from build123d import *

# Parameters (mm, degrees)
SKETCH1_W               = 297
SKETCH1_H               = 210
BOSS_EXTRUDE1_DEPTH     = 3
SKETCH2_OUTSIDE_W       = 371.752
SKETCH2_OUTSIDE_H       = 284.752
SKETCH2_OUTSIDE_R       = 1.5
LASER_CUT_PROFILE_DEPTH = 364.755412331


with BuildPart() as part:
    # Sketch1 → Boss-Extrude1 (new body)
    with BuildSketch(Plane(origin=(0, 0, 0), x_dir=(1, 0, 0), z_dir=(0, 1, 0))):
        with Locations((148.5, 105)):
            Rectangle(SKETCH1_W, SKETCH1_H)
    extrude(amount=BOSS_EXTRUDE1_DEPTH)

    # Sketch2 outside → Laser Cut Profile (cut, through all)
    # profile 1 of 14: a face of its own
    with BuildSketch(Plane(origin=(0, 3, 0), x_dir=(1, 0, 0), z_dir=(0, 1, 0))):
        with Locations((148.5, 105)):
            Rectangle(SKETCH2_OUTSIDE_W, SKETCH2_OUTSIDE_H)
        with BuildLine():
            Line((5, 2), (292, 2))
            ThreePointArc((292, 2), (294.121320344, 2.878679656), (295, 5))
            Line((295, 5), (295, 125))
            ThreePointArc((295, 125), (294.712859503, 126.280778403), (293.906404455, 127.316381241))
            Line((293.906404455, 127.316381241), (228.29357677, 181.316381241))
            ThreePointArc((228.29357677, 181.316381241), (227.399806572, 181.823928445), (226.387172315, 182))
            Line((226.387172315, 182), (70.612827685, 182))
            ThreePointArc((70.612827685, 182), (69.600193428, 181.823928445), (68.70642323, 181.316381241))
            Line((68.70642323, 181.316381241), (3.093595545, 127.316381241))
            ThreePointArc((3.093595545, 127.316381241), (2.287140497, 126.280778403), (2, 125))
            Line((2, 125), (2, 5))
            ThreePointArc((2, 5), (2.878679656, 2.878679656), (5, 2))
        make_face(mode=Mode.SUBTRACT)
    # profile 2 of 14: a face of its own
    with BuildSketch(Plane(origin=(0, 3, 0), x_dir=(1, 0, 0), z_dir=(0, 1, 0))):
        with Locations(Location((93.3, 92.8, 0), (0, 0, 270))):
            Circle(SKETCH2_OUTSIDE_R)
    # profile 3 of 14: a face of its own
    with BuildSketch(Plane(origin=(0, 3, 0), x_dir=(1, 0, 0), z_dir=(0, 1, 0))):
        with Locations(Location((141.2, 98.9, 0), (0, 0, 270))):
            Circle(SKETCH2_OUTSIDE_R)
    # profile 4 of 14: a face of its own
    with BuildSketch(Plane(origin=(0, 3, 0), x_dir=(1, 0, 0), z_dir=(0, 1, 0))):
        with Locations(Location((136.2, 68.95, 0), (0, 0, 270))):
            Circle(SKETCH2_OUTSIDE_R)
    # profile 5 of 14: a face of its own
    with BuildSketch(Plane(origin=(0, 3, 0), x_dir=(1, 0, 0), z_dir=(0, 1, 0))):
        with Locations(Location((108.5, 68.95, 0), (0, 0, 270))):
            Circle(SKETCH2_OUTSIDE_R)
    # profile 6 of 14: a face of its own
    with BuildSketch(Plane(origin=(0, 3, 0), x_dir=(1, 0, 0), z_dir=(0, 1, 0))):
        with Locations(Location((93.2, 18.35, 0), (0, 0, 270))):
            Circle(SKETCH2_OUTSIDE_R)
    # profile 7 of 14: a face of its own
    with BuildSketch(Plane(origin=(0, 3, 0), x_dir=(1, 0, 0), z_dir=(0, 1, 0))):
        with Locations(Location((141.2, 17.1, 0), (0, 0, 270))):
            Circle(SKETCH2_OUTSIDE_R)
    # profile 8 of 14: a face of its own
    with BuildSketch(Plane(origin=(0, 3, 0), x_dir=(1, 0, 0), z_dir=(0, 1, 0))):
        with Locations(Location((151.6, 18.4, 0), (0, 0, 270))):
            Circle(SKETCH2_OUTSIDE_R)
    # profile 9 of 14: a face of its own
    with BuildSketch(Plane(origin=(0, 3, 0), x_dir=(1, 0, 0), z_dir=(0, 1, 0))):
        with Locations(Location((166.65, 68.9, 0), (0, 0, 270))):
            Circle(SKETCH2_OUTSIDE_R)
    # profile 10 of 14: a face of its own
    with BuildSketch(Plane(origin=(0, 3, 0), x_dir=(1, 0, 0), z_dir=(0, 1, 0))):
        with Locations(Location((194.6, 68.9, 0), (0, 0, 270))):
            Circle(SKETCH2_OUTSIDE_R)
    # profile 11 of 14: a face of its own
    with BuildSketch(Plane(origin=(0, 3, 0), x_dir=(1, 0, 0), z_dir=(0, 1, 0))):
        with Locations(Location((83.275, 129.849046067, 0), (0, 0, 270))):
            Circle(SKETCH2_OUTSIDE_R)
    # profile 12 of 14: a face of its own
    with BuildSketch(Plane(origin=(0, 3, 0), x_dir=(1, 0, 0), z_dir=(0, 1, 0))):
        with Locations(Location((213.725, 129.849046067, 0), (0, 0, 270))):
            Circle(SKETCH2_OUTSIDE_R)
    # profile 13 of 14: a face of its own
    with BuildSketch(Plane(origin=(0, 3, 0), x_dir=(1, 0, 0), z_dir=(0, 1, 0))):
        with Locations(Location((83.275, 168.099046067, 0), (0, 0, 270))):
            Circle(SKETCH2_OUTSIDE_R)
    # profile 14 of 14: a face of its own
    with BuildSketch(Plane(origin=(0, 3, 0), x_dir=(1, 0, 0), z_dir=(0, 1, 0))):
        with Locations(Location((213.725, 168.099046067, 0), (0, 0, 270))):
            Circle(SKETCH2_OUTSIDE_R)
    extrude(amount=-LASER_CUT_PROFILE_DEPTH, mode=Mode.SUBTRACT)


solid = part.part
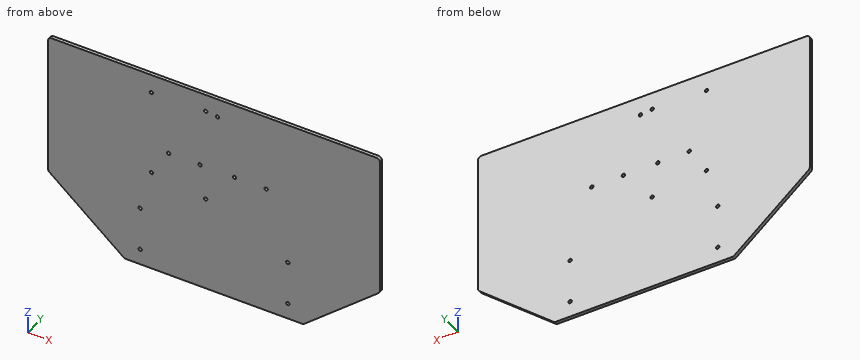
Build history of the part. All positions in model axes, mm. Round coordinates to 2 decimals unless told otherwise and drop trailing zeros. Write each loop counter-clockwise with the first axis right and the second up, starting at its lowest first coordinate (ties: lowest second). Pieces come first, ordered by that corner, then holes. Notation, with made-up numbers: (75, -8.5) -> (114, -8.5) arc R10 cw to (114, 1.5) -> close; hole circle Ø1 at (80, 84.5). An arc over 180 degrees is marked (long way). Use one line per item in the form item = value.
Q1. Band-saw the part on C-C, the plane z = -150. Write the cut outline in (x, y).
Conclusion:
outline = (30.66, 0) -> (266.34, 0) -> (266.34, 3) -> (30.66, 3) -> close
Q2. Band-saw the part on A-A, the plane y = 1.7. State how many separate pieces and enclosed holes the cut face has, then the cut area to 3 significant figures.
Conclusion:
separate_pieces = 1
enclosed_holes = 13
area = 48,900 mm²
Q3. Drop a flat-ended pin along its axis: P1, Ø1, axis at y = 0.5, z = -147.5, coming from the -X side. Give the stop position or say it passes through.
Conclusion:
P1 = 27.01
Q4. Drill centre lines: L1, parallel to Z at x = 93.3, y = 0.6; L2, parallel to Z at x = 83, y = 2.5; L3, parallel to X at y = 0.7, z = -92.8. Where is each one in solid material? Low to high.
Conclusion:
L1 = -182 to -94.3, -91.3 to -19.85, -16.85 to -2
L2 = -182 to -169.57, -166.62 to -131.32, -128.37 to -2
L3 = 2 to 91.8, 94.8 to 295
Q5. Band-saw the part on B-B, the plane x = 233. Write the cut outline in (y, z), then the cut area to 3 significant figures.
Conclusion:
outline = (0, -177.44) -> (3, -177.44) -> (3, -2) -> (0, -2) -> close
area = 526 mm²
